from build123d import *

# Parameters (mm, degrees)
BOSS_EXTRUDE1_DEPTH = 25
BOSS_EXTRUDE2_DEPTH = 15


with BuildPart() as part:
    # Sketch1 → Boss-Extrude1 (new body)
    with BuildSketch(Plane.XY):
        Polygon((0, 0), (0, 15), (15, 15), (15, 5), (30, 5), (30, 0), align=None)
    extrude(amount=BOSS_EXTRUDE1_DEPTH)

    # Sketch2 → Boss-Extrude2 (add)
    with BuildSketch(Plane(origin=(15, 0, 0), x_dir=(0, 0, -1), z_dir=(1, 0, 0))):
        Polygon((-25, 5), (0, 25), (0, 5), align=None)
    extrude(amount=BOSS_EXTRUDE2_DEPTH)


solid = part.part
Work out the finished part from the listing and answer in its coordinate system (mm). A direction names the side the tool comes from. Give positions to 0.01 mm unless a question says otherwise; leave off trailing zeros. Write each loop counter-clockwise with the first axis right and the second up, starting at its lowest first coordinate (ties: lowest second). Pieces come first, ordered by that corner, then holes. Notation, with made-up numbers: (70.25, 9.25) - (111.25, 9.25) arc R14 cw to (111.25, 30.25) - close; hole circle Ø9 at (52, 47). An arc over 180 degrees is marked (long way). One line per item, written item: value. Start each with the question number.
1. Find section D-D (z = 3.75). Write down the section's boundary in (x, y).
2. Consider probe 1 along Z at (x, y) = (17.75, 21); probe 2 along Y at (x, z) = (13.25, 13.5); probe 3 along X at (y, z) = (19.75, 1.75). Determine where each line is inside the solid, lowest interval first.
3. Find section B-B (y = 16). Write down the section's boundary in (x, z).
4. Given pin 1 (3 mm diameter, centred on x = 10.5, z = 20, fed in from +Y); pin 2 (10 mm diameter, centred on x = 25.5, z = 6, fed in from +Y), each flat-ended and moving along its own axis, determine where each tip first touches the part or whether it passes through.
5. Find section C-C (x = 23.25). Write down the section's boundary in (y, z).
6. For faces 1 (the flat face through (0, 7, 12)), 2 (the flat face through (15, 12, 21)), 3 (the flat face through (15, 18, 3)), determine the directions among +Z, -Z, +X, -X, +Y, -Y from which every point of the face is accessible in a straight line to the end or side of a thin tool.
7. For a pull along Y with two mould halves and no side action, classify faces 4 (the flat face through (15, 0, 12)), 5 (the flat face through (30, 10, 10)), 6 (the flat face through (22.395, 14.86, 12.675)) as +Y half, -Y half, draft (parallel to the pull), parting line (faces both ways), or undercut.
8. Find section A-A (z = 21.5). Write down the section's boundary in (x, y).
Geometry results:
1. outline: (0, 0) - (30, 0) - (30, 22) - (15, 22) - (15, 15) - (0, 15) - close
2. probe 1: 0 to 5
2. probe 2: 0 to 15
2. probe 3: 15 to 30
3. outline: (15, 0) - (30, 0) - (30, 11.25) - (15, 11.25) - close
4. pin 1: y = 15
4. pin 2: y = 24.2
5. outline: (0, 0) - (25, 0) - (5, 25) - (0, 25) - close
6. face 1: +Z, -Z, -X, +Y, -Y
6. face 2: +Z, +X, +Y
6. face 3: +Z, -Z, -X, +Y
7. face 4: -Y half
7. face 5: draft
7. face 6: +Y half
8. outline: (0, 0) - (30, 0) - (30, 7.8) - (15, 7.8) - (15, 15) - (0, 15) - close
